Geometry: final body of the model. Coordinates: model frame, mm. A direction names the side the tool comes from. Coordinates: 2 decimals unless noted, no trailing zeros. Order: outer loops, then holes, each group sorted by start corner. A loop starts at its lowest first (then second) coordinate and runs counter-clockwise, first axis right, second up. Notation, with made-up numbers: M 6.25,-40 L 35.25,-40 A30 cw 35.25,-8 Z; hole C 58,-8.75 d9. An arc over 180 degrees is marked long. One line per question, with ' | ' between items.
from build123d import *

# Parameters (mm, degrees)
SKETCH1_W           = 116
SKETCH1_H           = 83
SKETCH1_W_2         = 70
SKETCH1_H_2         = 77
SKETCH1_W_3         = 35
BOSS_EXTRUDE1_DEPTH = 30
SKETCH2_W           = 70
SKETCH2_H           = 77
SKETCH2_W_2         = 35
BOSS_EXTRUDE2_DEPTH = 3
SKETCH3_W           = 27
SKETCH3_H           = 5
CUT_EXTRUDE1_DEPTH  = 5
SKETCH5_R           = 5
CUT_EXTRUDE3_DEPTH  = 10
SKETCH6_R           = 1.75
CUT_EXTRUDE4_DEPTH  = 30
SKETCH7_W           = 9
SKETCH7_H           = 8
CUT_EXTRUDE5_DEPTH  = 10


with BuildPart() as part:
    # Sketch1 → Boss-Extrude1 (new body)
    with BuildSketch(Plane.XY):
        with Locations((-58, 41.5)):
            Rectangle(SKETCH1_W, SKETCH1_H)
        with Locations((-38, 41.5)):
            Rectangle(SKETCH1_W_2, SKETCH1_H_2, mode=Mode.SUBTRACT)
        with Locations((-95.5, 41.5)):
            Rectangle(SKETCH1_W_3, SKETCH1_H_2, mode=Mode.SUBTRACT)
    extrude(amount=BOSS_EXTRUDE1_DEPTH)

    # Sketch2 → Boss-Extrude2 (add)
    with BuildSketch(Plane(origin=(0, 0, 0), x_dir=(-1, 0, 0), z_dir=(0, 0, -1))):
        with Locations((38, 41.5)):
            Rectangle(SKETCH2_W, SKETCH2_H)
        with Locations((95.5, 41.5)):
            Rectangle(SKETCH2_W_2, SKETCH2_H)
    extrude(amount=-BOSS_EXTRUDE2_DEPTH)

    # Sketch3 → Cut-Extrude1 (cut)
    with BuildSketch(Plane(origin=(-73, 0, 0), x_dir=(0, 0, -1), z_dir=(1, 0, 0))):
        with Locations((-16.5, 77.5)):
            Rectangle(SKETCH3_W, SKETCH3_H)
    extrude(amount=-CUT_EXTRUDE1_DEPTH, mode=Mode.SUBTRACT)

    # Sketch5 → Cut-Extrude3 (cut)
    with BuildSketch(Plane(origin=(0, 0, 0), x_dir=(-1, 0, 0), z_dir=(0, -1, 0))):
        with Locations((12.5, -8)):
            Circle(SKETCH5_R)
    extrude(amount=-CUT_EXTRUDE3_DEPTH, mode=Mode.SUBTRACT)

    # Sketch6 → Cut-Extrude4 (cut)
    with BuildSketch(Plane.XY.offset(30)):
        with Locations((-75.5, 63)):
            Circle(SKETCH6_R)
        with Locations((-75.5, 20)):
            Circle(SKETCH6_R)
    extrude(amount=-CUT_EXTRUDE4_DEPTH, mode=Mode.SUBTRACT)

    # Sketch7 → Cut-Extrude5 (cut)
    with BuildSketch(Plane(origin=(0, 83, 0), x_dir=(1, 0, 0), z_dir=(0, 1, 0))):
        with Locations((-63.682179336, -26)):
            Rectangle(SKETCH7_W, SKETCH7_H)
    extrude(amount=-CUT_EXTRUDE5_DEPTH, mode=Mode.SUBTRACT)


solid = part.part
1. Pin query (flat end, axial travel): P1, Ø1.5, axis at x = -63, y = 81, coming from the +Z side; P2, Ø10, axis at x = -98.5, y = 11, coming from the +Z side. Return the tip coordinate at first contact, or that it passes through.
Response values:
P1: stops at z = 22 | P2: stops at z = 3
2. Material intervals for line 1 (Y direction, x = -75.5, z = 9); line 2 (X direction, y = 22, z = 13.5); line 3 (Y direction, x = -51, z = 7.5), sorted ascending. Write a range as [from, to].
Response values:
line 1: y = [0, 18.25], [21.75, 61.25], [64.75, 75], [80, 83] | line 2: x = [-116, -113], [-78, -73], [-3, 0] | line 3: y = [0, 3], [80, 83]
3. Section A-A, the plane x = -75.5. Output: boundary loops of the cut face in (y, z).
Response values:
outline: M 0,0 L 18.25,0 L 18.25,30 L 0,30 Z; M 21.75,0 L 61.25,0 L 61.25,30 L 21.75,30 Z; M 64.75,0 L 83,0 L 83,30 L 80,30 L 80,3 L 75,3 L 75,30 L 64.75,30 Z
4. Section C-C, the plane z = 11. Output: boundary loops of the cut face in (x, y).
Response values:
outline: M -116,0 L -16.5,0 L -16.5,3 L -73,3 L -73,75 L -78,75 L -78,3 L -113,3 L -113,80 L -3,80 L -3,3 L -8.5,3 L -8.5,0 L 0,0 L 0,83 L -116,83 Z; hole C -75.5,20 d3.5; hole C -75.5,63 d3.5
5. Section B-B, the plane y = 20. Output: boundary loops of the cut face in (x, z), and give its area (3 significant figures).
Response values:
outline: M -116,0 L -77.25,0 L -77.25,30 L -78,30 L -78,3 L -113,3 L -113,30 L -116,30 Z; M -73.75,0 L 0,0 L 0,30 L -3,30 L -3,3 L -73,3 L -73,30 L -73.75,30 Z | area: 540 mm^2
6. Access query for faces 4 (the face through (-59.182, 82, 26)), 5 (the face through (-113, 41, 16)), 6 (the face through (-73.883, 62.33, 15.21)), 7 (the face through (-17.27, 1.48, 6.5)). Directions: +Z, -Z, +X, -X, +Y, -Y. A direction counts if a zero-diameter tool reaches every point of the face in a straight line with its end or side. Return the directions, or none.
Response values:
face 4: +Z, +Y | face 5: +Z | face 6: +Z, -Z | face 7: -Y
7. Section D-D, the plane x = -10.5. Output: boundary loops of the cut face in (y, z), and give its area (3 significant figures).
Response values:
outline: M 0,0 L 83,0 L 83,30 L 80,30 L 80,3 L 3,3 L 3,3.42 L 0,3.42 Z; M 0,12.58 L 3,12.58 L 3,30 L 0,30 Z | area: 384 mm^2
8. Draft query along Y for faces 1 (the face through (-75, 39, 30)), 2 (the face through (-59, 83, 15)), 3 (the face through (-78, 38, 16)). Return one class per face: pulls with the +Y half, pulls with the -Y half, needs draft (parallel to the pull), parting line crosses it, or undercut.
Response values:
face 1: needs draft | face 2: pulls with the +Y half | face 3: undercut
